from build123d import *

# Parameters (mm, degrees)
SKETCH_1_W          = 1.8
SKETCH_1_H          = 8
EXTRUDE_1_DEPTH     = 20
SKETCH_3_R          = 0.7
CUT_EXTRUDE_1_DEPTH = 20
FILLET_1_R          = 1.5


with BuildPart() as part:
    # 草圖1 → 填料-伸長1 (new body)
    with BuildSketch(Plane(origin=(0, 0, 0), x_dir=(1, 0, 0), z_dir=(0, 1, 0))):
        Rectangle(SKETCH_1_W, SKETCH_1_H)
    extrude(amount=EXTRUDE_1_DEPTH)

    # 草圖3 → 除料-伸長1 (cut)
    with BuildSketch(Plane(origin=(0.9, 0, 0), x_dir=(0, 0, -1), z_dir=(1, 0, 0))):
        with Locations((-2.5, 18)):
            Circle(SKETCH_3_R)
        with Locations((-2.5, 15)):
            Circle(SKETCH_3_R)
        with Locations((-2.5, 12)):
            Circle(SKETCH_3_R)
        with Locations((-2.5, 9)):
            Circle(SKETCH_3_R)
        with Locations((-2.5, 6)):
            Circle(SKETCH_3_R)
        Polygon((-1.554314994, 20), (0.230558493, 17.700704895), (1.525082121, 12.032260524), (4, 5.822351238), (4, 20), align=None)
    extrude(amount=-CUT_EXTRUDE_1_DEPTH, mode=Mode.SUBTRACT)

    # 圓角1
    fillet_1_edges = [part.edges().sort_by_distance(p)[0] for p in [
        (0, 20, 1.554314994),
        (0, 12.032260524, -1.525082121),
        (0, 5.822351238, -4),
        (0, 17.700704895, -0.230558493),
        (0, 20, 4),
    ]]
    fillet(fillet_1_edges, radius=FILLET_1_R)


solid = part.part
Could you check a few things on this model? Use its own coordinates, in mm. Give positions to 0.01 mm unless a question says otherwise; leave off trailing zeros. Order: outer loops, then holes, each group sorted by start corner. A loop starts at its lowest first (then second) coordinate and runs counter-clockwise, first axis right, second up. Notation, with made-up numbers: (17, 43.5) -> (23, 43.5) arc R30 cw to (23, 78.5) -> close; hole circle Ø1 at (-18, -37). An arc over 180 degrees is marked (long way). Return JSON: item names as keys, results as strings.
1. I need wall thicknesses on line 1 (Y direction, x = 0.3, z = 2.5); line 2 (Y direction, x = -0.25, z = 0.25); line 3 (Z direction, x = -0.65, y = 16.75). Which ranges of each line are inside material? Lowest first, please. Write a range as from..to.
Answer list:
{"line 1": "y = 0..5.3, 6.7..8.3, 9.7..11.3, 12.7..14.3, 15.7..17.3, 18.7..20", "line 2": "y = 0..18.32", "line 3": "z = -0.45..4"}
2. Imagine slicing it at B-B on y = 15. List the corners of the cut face in (x, z) for me.
Answer list:
{"outline": "(-0.9, -0.85) -> (0.9, -0.85) -> (0.9, 1.8) -> (-0.9, 1.8) -> close; (-0.9, 3.2) -> (0.9, 3.2) -> (0.9, 4) -> (-0.9, 4) -> close"}
3. Imagine slicing it at A-A on x = -0.15. List the corners of the cut face in (y, z) for me, then the cut area to 3 significant figures.
Answer list:
{"outline": "(0, -4) -> (5.53, -4) arc R1.5 ccw to (6.09, -3.89) -> (11.92, -1.57) arc R1.5 cw to (12.15, -1.5) -> (17.38, -0.3) arc R1.5 ccw to (17.96, -0.03) -> (19.42, 1.1) arc R1.5 ccw to (20, 2.29) -> (20, 2.5) arc R1.5 ccw to (18.5, 4) -> (0, 4) -> close; hole circle Ø1.4 at (6, 2.5); hole circle Ø1.4 at (9, 2.5); hole circle Ø1.4 at (12, 2.5); hole circle Ø1.4 at (15, 2.5); hole circle Ø1.4 at (18, 2.5)", "area": "116 mm2"}
4. Imagine slicing it at D-D on y = 9. List the corners of the cut face in (x, z) for me.
Answer list:
{"outline": "(-0.9, -2.73) -> (0.9, -2.73) -> (0.9, 1.8) -> (-0.9, 1.8) -> close; (-0.9, 3.2) -> (0.9, 3.2) -> (0.9, 4) -> (-0.9, 4) -> close"}
5. For pin 1 Ø1 at (x, z) = (0, -0.5) entering from +Y, with a flat end and sliding along its axis, tell me the tip position at first contact or that it passes through.
Answer list:
{"pin 1": "stops at y = 18"}
6. Thinking about a two-plate mould opening in Y: for faces 1 (the flat face through (0, 3, -4)), 2 (the cylindrical face through (0.01, 6.59, 2.12)), 3 (the cylindrical face through (0.01, 19.57, 3.55)), which applies, pulls with the +Y half, pulls with the -Y half, needs draft (parallel to the pull), parting line crosses it, or undercut?
Answer list:
{"face 1": "needs draft", "face 2": "undercut", "face 3": "pulls with the +Y half"}
7. Imagine slicing it at C-C on z = 3. List the corners of the cut face in (x, y) for me, then the cut area to 3 significant figures.
Answer list:
{"outline": "(-0.9, 0) -> (0.9, 0) -> (0.9, 5.51) -> (-0.9, 5.51) -> close; (-0.9, 6.49) -> (0.9, 6.49) -> (0.9, 8.51) -> (-0.9, 8.51) -> close; (-0.9, 9.49) -> (0.9, 9.49) -> (0.9, 11.51) -> (-0.9, 11.51) -> close; (-0.9, 12.49) -> (0.9, 12.49) -> (0.9, 14.51) -> (-0.9, 14.51) -> close; (-0.9, 15.49) -> (0.9, 15.49) -> (0.9, 17.51) -> (-0.9, 17.51) -> close; (-0.9, 18.49) -> (0.9, 18.49) -> (0.9, 19.91) -> (-0.9, 19.91) -> close", "area": "27.0 mm2"}
